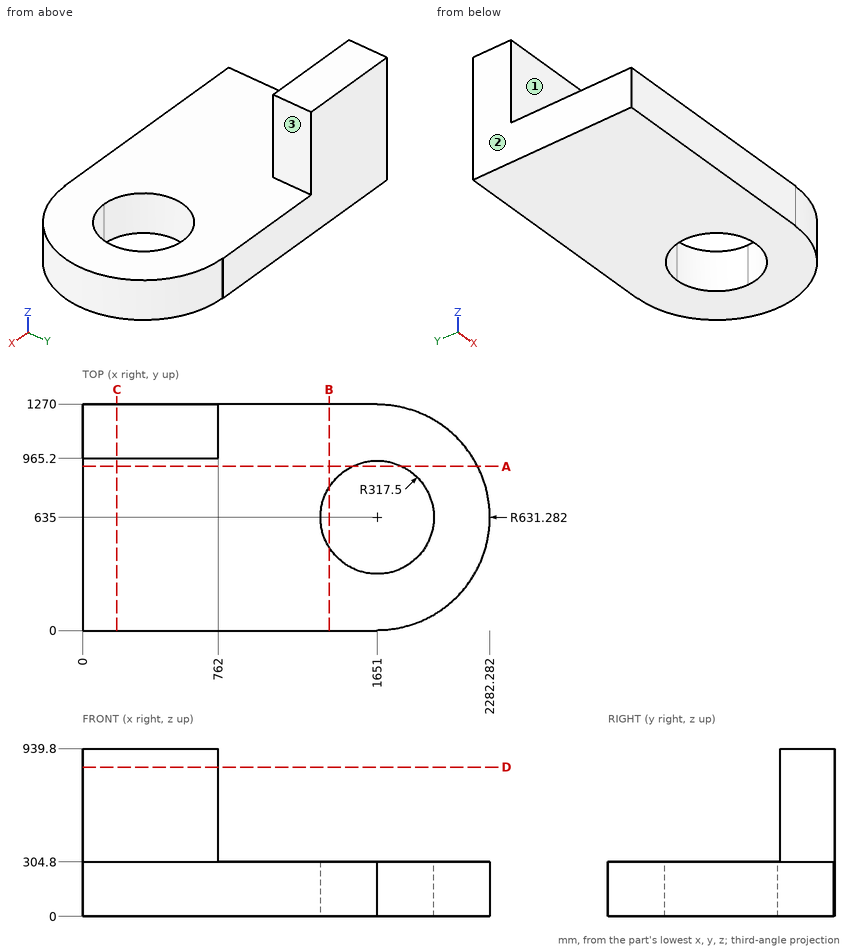
The drawing under review shows one solid part. Ordinate dimensions are in mm from its lowest x, y, z. A direction names the side the tool comes from. Round coordinates to 2 decimals unless told otherwise and drop trailing zeros. Loops run counter-clockwise (first coordinate to the right, second up) from the corner with the lowest first, then second, coordinate; pieces in that order, holes last. Notation, with made-up numbers: (-5.75, 36) - (49.25, 36) arc R24 cw to (49.25, 57) - close; hole circle Ø10 at (34, -6.75). An arc over 180 degrees is marked (long way). One line per question, with ' | ' between items.
1. We need section D-D, the plane z = 837. State the section outline as (x, y) points, and give its area (3 significant figures).
Results are:
outline: (0, 965.2) - (762, 965.2) - (762, 1270) - (0, 1270) - close | area: 232,000 mm²
2. We need section A-A, the plane y = 920. State the section outline as (x, z) points.
Results are:
outline: (0, 0) - (1511.07, 0) - (1511.07, 304.8) - (0, 304.8) - close; (1790.93, 0) - (2214.29, 0) - (2214.29, 304.8) - (1790.93, 304.8) - close
3. Clearance check with flat-ended pins moving along their axes: P1, Ø8, axis at x = 279.5, z = 728.5, coming from the -Y side; P2, Ø4, axis at y = 1.5, z = 144, coming from the +X side; P3, Ø4, axis at x = 1913, y = 312.5, coming from the +Z side. State where each tip first meets the part, or that it passes through.
Results are:
P1: stops at y = 965.2 | P2: stops at x = 1651 | P3: stops at z = 304.8
4. We need section C-C, the plane x = 192.5. State the section outline as (y, z) points.
Results are:
outline: (0, 0) - (1270, 0) - (1270, 939.8) - (965.2, 939.8) - (965.2, 304.8) - (0, 304.8) - close
5. We need section B-B, the plane x = 1382. State the section outline as (y, z) points, and give its area (3 significant figures).
Results are:
outline: (0, 0) - (466.34, 0) - (466.34, 304.8) - (0, 304.8) - close; (803.66, 0) - (1270, 0) - (1270, 304.8) - (803.66, 304.8) - close | area: 284,000 mm²
6. For L1, parallel to X at y = 623, z = 196.5; L2, parallel to Z at x = 823, y = 121; L3, parallel to Y at x = 625, z = 387.5, list the stretches that pass through material, from the lowest coordinate up. Write a range as [from, to].
Results are:
L1: x = [0, 1333.73], [1968.27, 2282.17] | L2: z = [0, 304.8] | L3: y = [965.2, 1270]
7. For the marked faces 1, 2 and 3, list the 3-axis set-ups (+Z, -Z, +X, -X, +Y, -Y) from which the entire face can be reached by the end or side of a thin tool; tool diameter is ignored.
Results are:
face 1: +Z, +X, -X, -Y | face 2: +Z, -Z, -X, +Y, -Y | face 3: +Z, +X, +Y, -Y
